Source: CAD feature listing. Evaluate the final solid. Frame: model axes, mm. A direction names the side the tool comes from. Give positions to 0.01 mm unless a question says otherwise; leave off trailing zeros. Order: outer loops, then holes, each group sorted by start corner. A loop starts at its lowest first (then second) coordinate and runs counter-clockwise, first axis right, second up. Notation, with made-up numbers: M 23,3.25 L 38,3.25 A20 cw 38,16.25 Z; hole C 38,1.5 d7. An arc over 180 degrees is marked long. Answer as a JSON object with one key per item and string values. Group by question number.
1. Material intervals for L1, parallel to Y at x = -1.15, z = 21.75; L2, parallel to Z at x = -0.2, y = 0.7; L3, parallel to Z at x = 1, y = -1.45, sorted ascending. Write a range as [from, to].
2. Pull-direction query (X, two-part tool) for faces 4 (the cylindrical face through (-0.585, -2.636, 21.09)), 5 (the flat face through (1.13, 0.64, 22.01)), 6 (the flat face through (-1.2, -1.2, 20)), 7 (the flat face through (1.12, -0.66, 22.01)); classes: +X half, -X half, draft (parallel to the pull), parting line (faces both ways), or undercut.
3. Section query B-B (z = 17.5). Output: boundary loops of the cut face in (x, y), plus the area to 3 significant figures.
4. Section query A-A (x = 0). Output: boundary loops of the cut face in (y, z).
5. Pin query (flat end, axial travel): P1, Ø1.5, axis at x = 1, z = 19, coming from the +Y side. Return the tip coordinate at first contact, or that it passes through.
6. Set-up query: faces 1 (the cylindrical face through (-1.5, 0.07, 10.39)), 2 (the flat face through (0, 0, 0)), 3 (the flat face through (0, 1.3, 22)). Return all of +Z, -Z, +X, -X, +Y, -Y with unobstructed straight access to the full face (end or side cutting, diameter ignored); none if empty.
from build123d import *

# Parameters (mm, degrees)
F3_DEPTH = 1.8
F4_R     = 0.75
F5_SIZE  = 0.5


with BuildPart() as f1:
    # F0 (on Front) → F1 (revolve)
    with BuildSketch(Plane.XZ):
        Polygon((0, 22.9), (0, 0), (1.5, 0), (1.5, 20), (2.7, 20), (2.7, 22.9), align=None)
    revolve(axis=Axis((0, 0, 11.45), (0, 0, 1)))

    # F2 (on face) → F3 (cut)
    with BuildSketch(Plane.XY.offset(22.9)):
        Polygon((0.750555, 1.3), (-0.750555, 1.3), (-1.501111, 0), (-0.750555, -1.3), (0.750555, -1.3), (1.501111, 0), align=None)
    extrude(amount=-F3_DEPTH, mode=Mode.SUBTRACT)

    # F4
    f4_edges = [f1.edges().sort_by_distance(p)[0] for p in [
        (-2.7, 0, 22.9),
    ]]
    fillet(f4_edges, radius=F4_R)

    # F5
    f5_edges = [f1.edges().sort_by_distance(p)[0] for p in [
        (-1.5, 0, 0),
    ]]
    chamfer(f5_edges, length=F5_SIZE)


solid = f1.part
Answer sheet:
{
 "1": {"L1": "[-2.44, -0.61], [0.61, 2.44]", "L2": "[0, 21.1]", "L3": "[20, 22.9]"},
 "2": {"face 4": "parting line", "face 5": "undercut", "face 6": "draft", "face 7": "undercut"},
 "3": {"outline": "C 0,0 d3", "area": "7.07 mm^2"},
 "4": {"outline": "M -2.7,20 L -1.5,20 L -1.5,0.5 L -1,0 L 1,0 L 1.5,0.5 L 1.5,20 L 2.7,20 L 2.7,22.15 A0.75 ccw 1.95,22.9 L 1.3,22.9 L 1.3,21.1 L -1.3,21.1 L -1.3,22.9 L -1.95,22.9 A0.75 ccw -2.7,22.15 Z"},
 "5": {"P1": "y = 1.48"},
 "6": {"face 1": "-Z", "face 2": "-Z, +X, -X, +Y, -Y", "face 3": "+Z"}
}
